Build history of the part. All positions in model axes, mm. Round coordinates to 2 decimals unless told otherwise and drop trailing zeros. Write each loop counter-clockwise with the first axis right and the second up, starting at its lowest first coordinate (ties: lowest second). Pieces come first, ordered by that corner, then holes. Notation, with made-up numbers: (85.25, 69) -> (124.25, 69) arc R29 ccw to (124.25, 94) -> close; hole circle Ø2 at (68.25, 64). An arc over 180 degrees is marked (long way). Return JSON: item names as keys, results as strings.
Solid Edge part; units mm, degrees
sketch "Sketch1" plane through (0, 0, 0) normal (0, -1, 0) x (1, 0, 0)
  line L0 (-27.5, -5) -> (27.5, -5)
  arc A0 (27.5, -5) -> (27.5, 5) centre (27.5, 0) ccw
  line L1 (27.5, 5) -> (-27.5, 5)
  arc A1 (-27.5, -5) -> (-27.5, 5) centre (-27.5, 0) cw
  dimension "D1" = 27.5
  dimension "D2" = 27.5
extrude "Ajout_matière_1" add sketch "Sketch1" along normal blind 3
sketch "Sketch2" plane through (0, -3, 0) normal (0, -1, 0) x (1, 0, 0)
  circle A0 centre (-7.5, 0) radius 0.85
  circle A1 centre (-27.5, 0) radius 1.075
  circle A2 centre (27.5, 0) radius 0.85
extrude "Enlèvement_matière_1" cut sketch "Sketch2" against normal blind 215.5447
properties part number "16" material "MDF 3mm"
Q1. Two-plate mould, pull along Z, no slides. Class faces 1 (the cylindrical face through (26.65, -1.52, 0.04)), 2 (the flat face through (0, -1, 5)), 3 (the flat face through (0, 0, 0)): +Z half, -Z half, draft (parallel to the pull), parting line (faces both ways), or undercut.
Verdict:
{"face 1": "undercut", "face 2": "+Z half", "face 3": "draft"}
Q2. Wall check: L1, parallel to X at y = -2.5, z = 0.5; L2, parallel to X at y = -2.4, z = 0.25; L3, parallel to Z at x = -27.5, y = -1.5 (3 decimals). Give the ranges that are in metal, low to high.
Verdict:
{"L1": "x = -32.47 to -28.45, -26.55 to -8.19, -6.81 to 26.81, 28.19 to 32.47", "L2": "x = -32.49 to -28.55, -26.45 to -8.31, -6.69 to 26.69, 28.31 to 32.49", "L3": "z = -5 to -1.075, 1.075 to 5"}
Q3. Saw through at D-D on z = 4. List the corners of the cut face in (x, y).
Verdict:
{"outline": "(-30.5, -3) -> (30.5, -3) -> (30.5, 0) -> (-30.5, 0) -> close"}
Q4. Pin check, flat tip, straight feed: pin 1 Ø1.5 at (x, z) = (-7.5, 0) entering from -Y. Stop position of the tip, or through.
Verdict:
{"pin 1": "passes through"}
Q5. Saw through at A-A on z = 0. List the corners of the cut face in (x, y) (3 decimals), then the cut area to 3 significant figures.
Verdict:
{"outline": "(-32.5, -3) -> (-28.575, -3) -> (-28.575, 0) -> (-32.5, 0) -> close; (-26.425, -3) -> (-8.35, -3) -> (-8.35, 0) -> (-26.425, 0) -> close; (-6.65, -3) -> (26.65, -3) -> (26.65, 0) -> (-6.65, 0) -> close; (28.35, -3) -> (32.5, -3) -> (32.5, 0) -> (28.35, 0) -> close", "area": "178 mm²"}
Q6. Saw through at B-B on x = -7.5. List the corners of the cut face in (y, z).
Verdict:
{"outline": "(-3, -5) -> (0, -5) -> (0, -0.85) -> (-3, -0.85) -> close; (-3, 0.85) -> (0, 0.85) -> (0, 5) -> (-3, 5) -> close"}
Q7. Saw through at C-C on y = -0.7. List the corners of the cut face in (x, z) (3 decimals), then the cut area to 3 significant figures.
Verdict:
{"outline": "(-27.5, -5) -> (27.5, -5) arc R5 ccw to (27.5, 5) -> (-27.5, 5) arc R5 ccw to start; hole circle Ø2.15 at (-27.5, 0); hole circle Ø1.7 at (-7.5, 0); hole circle Ø1.7 at (27.5, 0)", "area": "620 mm²"}
